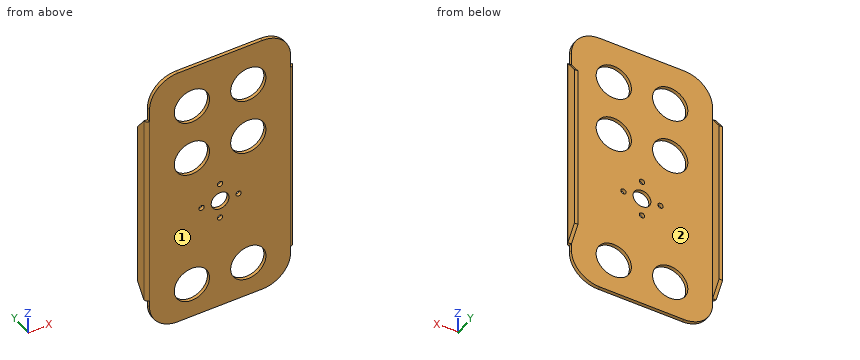
from build123d import *

# Parameters (mm, degrees)
SKETCH1_R               = 7.9375
SKETCH1_R_2             = 4.0005
SKETCH1_R_3             = 1.1938
EXTRUDE1_DEPTH          = 1.524
EXTRUDE2_DEPTH          = 6.35
CUT_EXTRUDE1_DEPTH      = 34.3502
CUT_EXTRUDE1_DEPTH_BACK = 34.3502
FILLET1_R               = 1.5875


with BuildPart() as part:
    # Sketch1 → Extrude1 (new body)
    with BuildSketch(Plane(origin=(0, 0, 0), x_dir=(1, 0, 0), z_dir=(0, 1, 0))):
        with BuildLine():
            Line((-31.75, -3.2004), (-31.75, -58.7756))
            ThreePointArc((-31.75, -58.7756), (-28.030256121, -67.755856121), (-19.05, -71.4756))
            Line((-19.05, -71.4756), (19.05, -71.4756))
            ThreePointArc((19.05, -71.4756), (28.030256121, -67.755856121), (31.75, -58.7756))
            Line((31.75, -58.7756), (31.75, -3.2004))
            Line((31.75, -3.2004), (31.75, 39.2684))
            ThreePointArc((31.75, 39.2684), (28.030256121, 48.248656121), (19.05, 51.9684))
            Line((19.05, 51.9684), (12.7, 51.9684))
            Line((12.7, 51.9684), (-12.7, 51.9684))
            Line((-12.7, 51.9684), (-19.05, 51.9684))
            ThreePointArc((-19.05, 51.9684), (-28.030256121, 48.248656121), (-31.75, 39.2684))
            Line((-31.75, 39.2684), (-31.75, -3.2004))
        make_face()
        with Locations(Location((-12.7, -52.4002, 0), (0, 0, 270))):  # turned: the seam where the file's is
            Circle(SKETCH1_R, mode=Mode.SUBTRACT)
        with Locations(Location((-12.7, 36.0934, 0), (0, 0, 270))):  # turned: the seam where the file's is
            Circle(SKETCH1_R, mode=Mode.SUBTRACT)
        with Locations(Location((12.7, -52.4002, 0), (0, 0, 270))):  # turned: the seam where the file's is
            Circle(SKETCH1_R, mode=Mode.SUBTRACT)
        with Locations(Location((12.7, -26.5938, 0), (0, 0, 270))):  # turned: the seam where the file's is
            Circle(SKETCH1_R, mode=Mode.SUBTRACT)
        with Locations(Location((12.7, 36.0934, 0), (0, 0, 270))):  # turned: the seam where the file's is
            Circle(SKETCH1_R, mode=Mode.SUBTRACT)
        with Locations(Location((0, 0, 0), (0, 0, 270))):  # turned: the seam where the file's is
            Circle(SKETCH1_R_2, mode=Mode.SUBTRACT)
        with Locations(Location((8.3312, 0, 0), (0, 0, 270))):  # turned: the seam where the file's is
            Circle(SKETCH1_R_3, mode=Mode.SUBTRACT)
        with Locations(Location((0, -8.3312, 0), (0, 0, 270))):  # turned: the seam where the file's is
            Circle(SKETCH1_R_3, mode=Mode.SUBTRACT)
        with Locations(Location((0, 8.3312, 0), (0, 0, 270))):  # turned: the seam where the file's is
            Circle(SKETCH1_R_3, mode=Mode.SUBTRACT)
        with Locations(Location((-8.3312, 0, 0), (0, 0, 270))):  # turned: the seam where the file's is
            Circle(SKETCH1_R_3, mode=Mode.SUBTRACT)
        with Locations(Location((-12.7, -26.5938, 0), (0, 0, 270))):  # turned: the seam where the file's is
            Circle(SKETCH1_R, mode=Mode.SUBTRACT)
    extrude(amount=EXTRUDE1_DEPTH)

    # Sketch1_3 → Extrude2 (add)
    with BuildSketch(Plane(origin=(0, 0, 0), x_dir=(1, 0, 0), z_dir=(0, 1, 0))):
        Polygon((31.75, 36.0934), (31.75, -3.2004), (31.75, -52.8066), (33.3502, -52.8066), (33.3502, 36.0934), align=None)
        Polygon((-33.3502, -52.8066), (-31.75, -52.8066), (-31.75, -3.2004), (-31.75, 36.0934), (-33.3502, 36.0934), align=None)
    extrude(amount=EXTRUDE2_DEPTH)

    # Sketch2 → Cut-Extrude1 (cut, two sides)
    with BuildSketch(Plane(origin=(0, 0, 0), x_dir=(0, 0, -1), z_dir=(1, 0, 0))) as cut_extrude1_sk:
        Polygon((-52.8066, 1.524), (-46.4566, 6.35), (-52.8066, 6.35), align=None)
        Polygon((36.0934, 6.35), (36.0934, 1.524), (29.7434, 6.35), align=None)
    extrude(amount=CUT_EXTRUDE1_DEPTH, mode=Mode.SUBTRACT)
    extrude(cut_extrude1_sk.sketch, amount=-CUT_EXTRUDE1_DEPTH_BACK, mode=Mode.SUBTRACT)

    # Fillet1
    fillet1_edges = [part.edges().sort_by_distance(p)[0] for p in [
        (33.3502, 0, 8.3566),
        (-33.3502, 0, 8.3566),
    ]]
    fillet(fillet1_edges, radius=FILLET1_R)


solid = part.part
Can you work these out from the model? Positions are in its coordinate system, mm. Face numbers are marked on the shaded views. Round coordinates to 2 decimals unless told otherwise and drop trailing zeros. Write each loop counter-clockwise with the first axis right and the second up, starting at its lowest first coordinate (ties: lowest second). Pieces come first, ordered by that corner, then holes. Notation, with made-up numbers: (-30, -3) -> (-19, -3) arc R23 cw to (-19, 8) -> close; hole circle Ø10 at (-19.75, 62.25). An arc over 180 degrees is marked (long way). One line per question, with ' | ' between items. Start each with the question number.
1) If we mould it in two halves opening along X, with no side actions, what happens to the marked faces 1 and 2? For each: released by +X, released by -X, zero draft, split by the parting line, or undercut.
2) Suppose I cut it at B-B on z = 0. Count the separate pieces of the cut face and the enclosed holes in it, then the cut area to 3 significant figures.
3) I'm going to push flat-ended pins straight in: P1, Ø7, axis at x = 0, z = 0, coming from the +Y side; P2, Ø1.2, axis at x = 32.5, y = 0.5, coming from the -Z side; P3, Ø10, axis at x = -9.5, z = -20.5, coming from the +Y side; P4, Ø0.5, axis at y = 1, z = -37.5, coming from the +X side. Where does each tip first touch, or does it pass through?
4) Suppose I cut it at A-A on x = 12.7. Write out the boundary of the cut face in (y, z).
5) Suppose I cut it at C-C on y = 4.5. Write out the boundary of the cut face in (x, z).
6) I need wall thicknesses on line 1 (X direction, y = 2, z = -14.5); line 2 (Y direction, x = -12, z = 1); line 3 (Z direction, x = -5.5, y = 1). Which ranges of each line are inside material? Lowest first, please. Write a range as [from, to].
Return value:
1) face 1: zero draft | face 2: undercut
2) separate pieces: 4 | enclosed holes: 0 | area: 96.5 mm2
3) P1: passes through | P2: stops at z = -36.09 | P3: stops at y = 1.52 | P4: stops at x = 31.75
4) outline: (0, -51.97) -> (1.52, -51.97) -> (1.52, -44.03) -> (0, -44.03) -> close; (0, -28.16) -> (1.52, -28.16) -> (1.52, 18.66) -> (0, 18.66) -> close; (0, 34.53) -> (1.52, 34.53) -> (1.52, 44.46) -> (0, 44.46) -> close; (0, 60.34) -> (1.52, 60.34) -> (1.52, 71.48) -> (0, 71.48) -> close
5) outline: (-33.35, -32.18) -> (-31.75, -32.18) -> (-31.75, 48.89) -> (-33.35, 48.89) -> close; (31.75, -32.18) -> (33.35, -32.18) -> (33.35, 48.89) -> (31.75, 48.89) -> close
6) line 1: x = [-33.35, -31.75], [31.75, 33.35] | line 2: y = [0, 1.52] | line 3: z = [-51.97, -39.43], [-32.75, 23.25], [29.94, 49.06], [55.74, 71.48]
